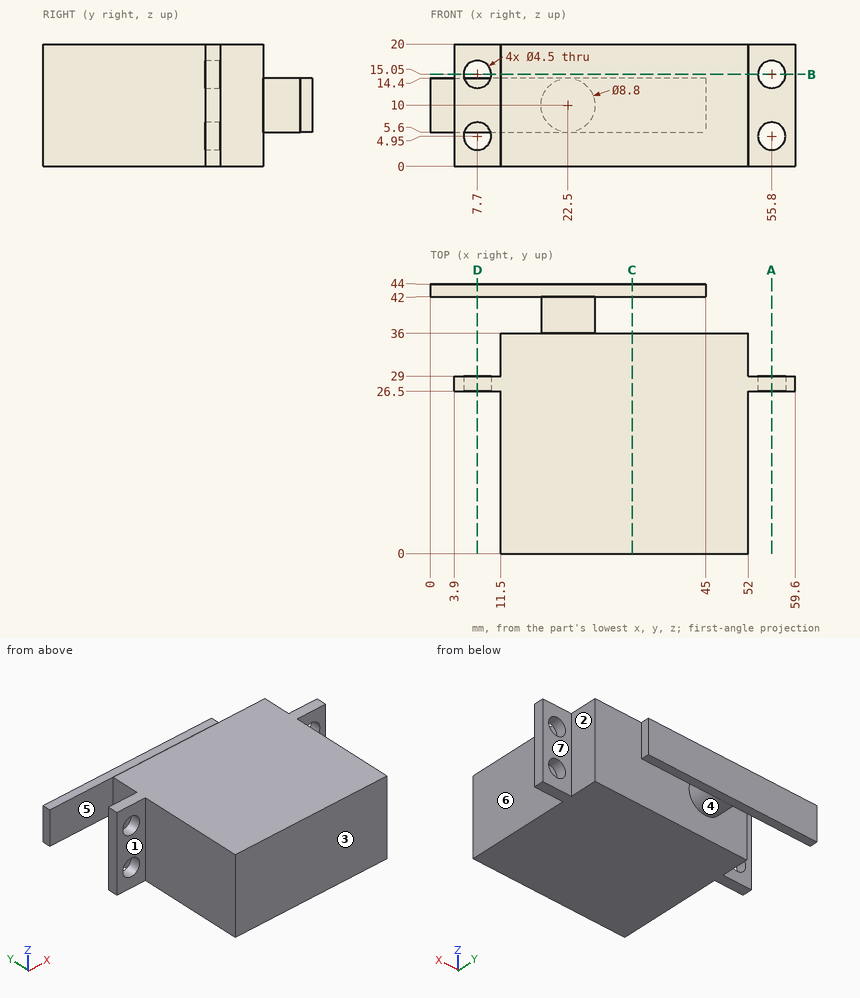
Answer from the drawing. Dimensions are ordinates in mm from the lowest x, y and z of the part. A direction names the side the tool comes from. Give positions to 0.01 mm unless a question says otherwise; leave off trailing zeros. Write each loop counter-clockwise with the first axis right and the second up, starting at its lowest first coordinate (ties: lowest second). Pieces come first, ordered by that corner, then holes. Notation, with made-up numbers: (45.25, 74) -> (98.25, 74) arc R8 cw to (98.25, 80) -> close; hole circle Ø5 at (55, 13.5). An arc over 180 degrees is marked (long way). Use a Markdown table: item, result.
(1) For the marked faces 1, 2 and 3, determine the directions among +Z, -Z, +X, -X, +Y, -Y from which every point of the face is accessible in a straight line to the end or side of a thin tool.
Return value:
| item | result |
|---|---|
| face 1 | +Z, -Z, -X, -Y |
| face 2 | +Z, -Z, +X, +Y |
| face 3 | +Z, -Z, +X, -X, -Y |
(2) Determine the mould class of the marked faces 4, 5, 6 and 7 for opening direction Y: released by +Y, released by -Y, zero draft, split by the parting line, or undercut.
Return value:
| item | result |
|---|---|
| face 4 | undercut |
| face 5 | undercut |
| face 6 | zero draft |
| face 7 | released by +Y |
(3) Section B-B, the plane z = 15.05 is taken. Determine the outline of the cut face in (x, y).
Return value:
| item | result |
|---|---|
| outline | (3.9, 26.5) -> (5.45, 26.5) -> (5.45, 29) -> (3.9, 29) -> close; (9.95, 26.5) -> (11.5, 26.5) -> (11.5, 0) -> (52, 0) -> (52, 26.5) -> (53.55, 26.5) -> (53.55, 29) -> (52, 29) -> (52, 36) -> (11.5, 36) -> (11.5, 29) -> (9.95, 29) -> close; (58.05, 26.5) -> (59.6, 26.5) -> (59.6, 29) -> (58.05, 29) -> close |
(4) Section D-D, the plane x = 7.7 is taken. Determine the outline of the cut face in (y, z), then the cut area to 3 significant figures.
Return value:
| item | result |
|---|---|
| outline | (26.5, 0) -> (29, 0) -> (29, 2.7) -> (26.5, 2.7) -> close; (26.5, 7.2) -> (29, 7.2) -> (29, 12.8) -> (26.5, 12.8) -> close; (26.5, 17.3) -> (29, 17.3) -> (29, 20) -> (26.5, 20) -> close; (42, 5.6) -> (44, 5.6) -> (44, 14.4) -> (42, 14.4) -> close |
| area | 45.1 mm2 |
(5) Section C-C, the plane x = 33 is taken. Determine the outline of the cut face in (y, z), then the cut area to 3 significant figures.
Return value:
| item | result |
|---|---|
| outline | (0, 0) -> (36, 0) -> (36, 20) -> (0, 20) -> close; (42, 5.6) -> (44, 5.6) -> (44, 14.4) -> (42, 14.4) -> close |
| area | 738 mm2 |
(6) Section A-A, the plane x = 55.8 is taken. Determine the outline of the cut face in (y, z), then the cut area to 3 significant figures.
Return value:
| item | result |
|---|---|
| outline | (26.5, 0) -> (29, 0) -> (29, 2.7) -> (26.5, 2.7) -> close; (26.5, 7.2) -> (29, 7.2) -> (29, 12.8) -> (26.5, 12.8) -> close; (26.5, 17.3) -> (29, 17.3) -> (29, 20) -> (26.5, 20) -> close |
| area | 27.5 mm2 |
(7) Find the intervals of material crossed by probe 1 along X at (y, z) = (28.25, 15.05); probe 2 along Y at (x, z) = (6.5, 8.75); probe 3 along Z at (x, y) = (55, 27), in increasing order. Write a range as from..to.
Return value:
| item | result |
|---|---|
| probe 1 | 3.9..5.45, 9.95..53.55, 58.05..59.6 |
| probe 2 | 26.5..29, 42..44 |
| probe 3 | 0..2.85, 7.05..12.95, 17.15..20 |
(8) Flat-ended cylindrical pins translate along their axes: P1, Ø8, axis at x = 19, y = 20, coming from the -Z side; P2, Ø6, axis at x = 57, z = 12.5, coming from the +Y side; P3, Ø3, axis at x = 50.5, z = 9, coming from the +Y side; P4, Ø1.6, axis at x = 24.5, y = 43, coming from the -Z side. Find the tip coordinate at first contact, or state that the pin passes through.
Return value:
| item | result |
|---|---|
| P1 | z = 0 |
| P2 | y = 29 |
| P3 | y = 36 |
| P4 | z = 5.6 |
